```python
from build123d import *

# Parameters (mm, degrees)
EXTRUDE_1_DEPTH = 1.5
SKETCH_2_R      = 2
EXTRUDE_2_DEPTH = 5


with BuildPart() as part:
    # 草图1 → 凸台-拉伸1 (new body)
    with BuildSketch(Plane(origin=(0, 0, 0), x_dir=(1, 0, 0), z_dir=(0, 1, 0))):
        Polygon((5.22625186, 0), (3.69551813, 3.69551813), (0, 5.22625186), (-3.69551813, 3.69551813), (-5.22625186, 0), (-3.69551813, -3.69551813), (0, -5.22625186), (3.69551813, -3.69551813), align=None)
    extrude(amount=EXTRUDE_1_DEPTH)

    # 草图2 → 凸台-拉伸2 (add)
    with BuildSketch(Plane(origin=(0, 1.5, 0), x_dir=(1, 0, 0), z_dir=(0, 1, 0))):
        with Locations(Location((0, 0, 0), (0, 0, 270))):
            Circle(SKETCH_2_R)
    extrude(amount=EXTRUDE_2_DEPTH)


solid = part.part
```
Could you check a few things on this model? Use its own coordinates, in mm. A direction names the side the tool comes from. Coordinates: 2 decimals unless noted, no trailing zeros. Write each loop counter-clockwise with the first axis right and the second up, starting at its lowest first coordinate (ties: lowest second). Pieces come first, ordered by that corner, then holes. Notation, with made-up numbers: (15.25, 44.5) -> (66.25, 44.5) arc R14 ccw to (66.25, 51.5) -> close; hole circle Ø2 at (3.5, -11). An arc over 180 degrees is marked (long way). Write item = value, one per line. Start each with the question number.
(1) I need wall thicknesses on line 1 (Y direction, x = 2.5, z = 3.75); line 2 (X direction, y = 3.75, z = -1.5); line 3 (Z direction, x = 1.25, y = 2.75). Which ranges of each line are inside material? Lowest first, please. Write a range as [from, to].
(2) I want a section at A-A (x = 1.25). Please give me the cut outline in (y, z), plus the area to 3 significant figures.
(3) Which directions (+Z, -Z, +X, -X, +Y, -Y) give clear straight access to the entire face, cutting with the end or side of a thin tool? Please do faces 1 (the face through (-0.1, 1.5, 2.2)), 2 (the face through (-1.822, 0.74, -4.472)).
(4) I want a section at C-C (x = -1.5). Please give me the cut outline in (y, z).
(5) Will these pins go through, and if not, where does the flat tip stop? pin 1 (2 mm diameter, centred on x = -1.5, z = 3.5, fed in from +Y); pin 2 (3 mm diameter, centred on y = 5.5, z = 3, fed in from -X).
(6) I want a section at B-B (y = 5.75). Please give me the cut outline in (x, z), plus the area to 3 significant figures.
(7) I want a section at D-D (x = 4). Please give me the cut outline in (y, z), plus the area to 3 significant figures.
Result set:
q1.line_1 = [0, 1.5]
q1.line_2 = [-1.32, 1.32]
q1.line_3 = [-1.56, 1.56]
q2.outline = (0, -4.71) -> (1.5, -4.71) -> (1.5, -1.56) -> (6.5, -1.56) -> (6.5, 1.56) -> (1.5, 1.56) -> (1.5, 4.71) -> (0, 4.71) -> close
q2.area = 29.7 mm2
q3.face_1 = +Y
q3.face_2 = -Z, -X, +Y, -Y
q4.outline = (0, -4.6) -> (1.5, -4.6) -> (1.5, -1.32) -> (6.5, -1.32) -> (6.5, 1.32) -> (1.5, 1.32) -> (1.5, 4.6) -> (0, 4.6) -> close
q5.pin_1 = 1.5
q5.pin_2 = -1.32
q6.outline = circle Ø4 at (0, 0)
q6.area = 12.6 mm2
q7.outline = (0, -2.96) -> (1.5, -2.96) -> (1.5, 2.96) -> (0, 2.96) -> close
q7.area = 8.88 mm2
